Autodesk Inventor part; units mm, degrees
ref_plane "YZ Plane" through (0, 0, 0) normal (1, 0, 0) x (0, 1, 0)
ref_plane "XZ Plane" through (0, 0, 0) normal (0, 1, 0) x (-1, 0, 0)
ref_plane "XY Plane" through (0, 0, 0) normal (0, 0, 1) x (1, 0, 0)
sketch "Sketch1" plane through (0, 0, 0) normal (1, 0, 0) x (0, 1, 0)
  line L0 (0, 0) -> (25, 0)
  line L1 (25, 0) -> (25, -35)
  line L2 (25, -35) -> (0, -35)
  line L3 (0, -35) -> (0, 0)
  circle A0 centre (19, -7.5) radius 2
  circle A1 centre (19, -27.5) radius 2
  dimension "d0" = 25
  dimension "d1" = 35
  dimension "d5" = 4
  dimension "d6" = 4
extrude "Extrusion1" add sketch "Sketch1" along normal blind 6
sketch "Sketch2" plane through (6, 0, 0) normal (1, 0, 0) x (0, 0, -1)
  line L0 (0, 0) -> (7, 0)
  line L1 (7, 0) -> (7, 6)
  line L2 (7, 6) -> (0, 6)
  line L3 (0, 6) -> (0, 0)
  dimension "d9" = 7
  dimension "d10" = 6
extrude "Extrusion2" cut sketch "Sketch2" against normal blind 6
pattern_linear "Rectangular Pattern1" count 3 spacing 14 along (0, 0, -1) of "Extrusion2"
properties part number "g_mount 1"
Could you check a few things on this model? Use its own coordinates, in mm. A direction names the side the tool comes from. Round coordinates to 2 decimals unless told otherwise and drop trailing zeros. Loops run counter-clockwise (first coordinate to the right, second up) from the corner with the lowest first, then second, coordinate; pieces in that order, holes last.
Q1. I want a section at A-A (y = 4.25). Write out the boundary of the cut face in (x, z), and give its area (3 significant figures).
Q2. Thinking about a two-plate mould opening in Z: for faces 4 (the cylindrical face through (2.958, 18.566, -25.548)), 5 (the flat face through (3, 6, -32)), 6 (the flat face through (3, 3, -28)), which applies, pulls with the +Z half, pulls with the -Z half, needs draft (parallel to the pull), parting line crosses it, or undercut?
Q3. I want a section at C-C (x = 4.6). Write out the boundary of the cut face in (y, z), and give its area (3 significant figures).
Q4. I want a section at B-B (z = -27.5). Write out the boundary of the cut face in (x, y), and give its area (3 significant figures).
Q5. For P1, Ø3, axis at x = 4, z = -30, coming from the -Y side; P2, Ø2.5, axis at y = 19, z = -7.5, coming from the +X side; P3, Ø1, axis at x = 2.5, y = 4, coming from the +Z side; P4, Ø3, axis at x = 3, y = 3.5, coming from the -Z side, each with a flat end and sliding along its axis, tell me the tip position at first contact or that it passes through.
Q6. I want a section at D-D (y = 19). Write out the boundary of the cut face in (x, z), and give its area (3 significant figures).
Q7. Please list where these lines run through material, in increasing order: L1, parallel to Z at x = 3.8, y = 19; L2, parallel to Z at x = 5.7, y = 1.5; L3, parallel to Z at x = 0.8, y = 20.5.
Q8. On a 3-axis mill with a long thin cutter (end or side, diameter ignored), from which of +Z, -Z, +X, -X, +Y, -Y can I reach the whole of each face in a straight line? I mean faces 1 (the flat face through (3, 3, -7)), 2 (the flat face through (3, 15, 0)), 3 (the flat face through (3, 3, -21)). Say none if no direction works.
Answer below:
1. outline: (0, -28) - (6, -28) - (6, -21) - (0, -21) - close; (0, -14) - (6, -14) - (6, -7) - (0, -7) - close
1. area: 84.0 mm2
2. face 4: undercut
2. face 5: needs draft
2. face 6: pulls with the -Z half
3. outline: (0, -28) - (6, -28) - (6, -35) - (25, -35) - (25, 0) - (6, 0) - (6, -7) - (0, -7) - (0, -14) - (6, -14) - (6, -21) - (0, -21) - close; hole circle Ø4 at (19, -27.5); hole circle Ø4 at (19, -7.5)
3. area: 724 mm2
4. outline: (0, 0) - (6, 0) - (6, 17) - (0, 17) - close; (0, 21) - (6, 21) - (6, 25) - (0, 25) - close
4. area: 126 mm2
5. P1: stops at y = 6
5. P2: passes through
5. P3: stops at z = -7
5. P4: stops at z = -28
6. outline: (0, -35) - (6, -35) - (6, -29.5) - (0, -29.5) - close; (0, -25.5) - (6, -25.5) - (6, -9.5) - (0, -9.5) - close; (0, -5.5) - (6, -5.5) - (6, 0) - (0, 0) - close
6. area: 162 mm2
7. L1: z = -35 to -29.5, -25.5 to -9.5, -5.5 to 0
7. L2: z = -28 to -21, -14 to -7
7. L3: z = -35 to -28.82, -26.18 to -8.82, -6.18 to 0
8. face 1: +Z, +X, -X, -Y
8. face 2: +Z, +X, -X, +Y, -Y
8. face 3: +X, -X, -Y
